Here's how the part is built. I have some questions about the finished solid (model axes, mm). Coordinates: 2 decimals unless noted, no trailing zeros. Loops run counter-clockwise (first coordinate to the right, second up) from the corner with the lowest first, then second, coordinate; pieces in that order, holes last. Notation, with made-up numbers: (-11.5, 55) - (25.5, 55) arc R11 cw to (25.5, 63) - close; hole circle Ø4 at (35, 77). An arc over 180 degrees is marked (long way). Use a Markdown table: item, result.
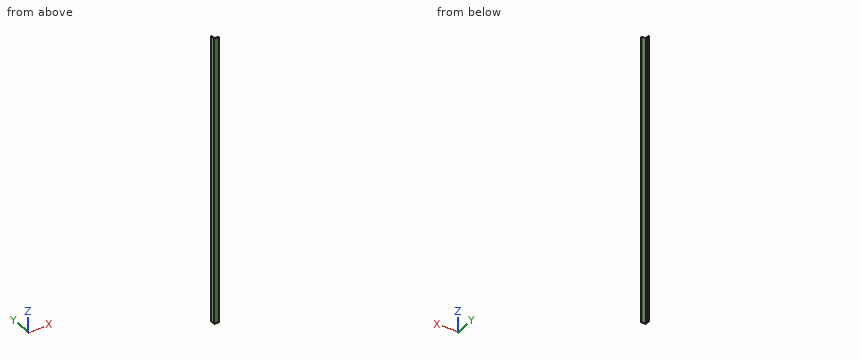
Autodesk Inventor part; units mm, degrees
ref_plane "Plano inicial" through (0, 0, 0) normal (0, 0, 1) x (1, 0, 0)
ref_plane "Plano final" through (0, 0, 2400) normal (0, 0, 1) x (1, 0, 0)
ref_plane "Plano de trabajo4" through (4.8672, 4.8672, 1401) normal (0, 0, 1) x (1, 0, 0)
ref_plane "Plano inicial" through (0, 0, 0) normal (0, 0, 1) x (1, 0, 0)
ref_plane "Plano final" through (0, 0, 2400) normal (0, 0, 1) x (1, 0, 0)
sketch "Boceto" plane through (0, 0, 0) normal (0, 0, 1) x (1, 0, 0)
  line L0 (38.1, 0) -> (0, 0)
  line L1 (0, 0) -> (0, 38.1)
  line L2 (0, 38.1) -> (2.4765, 38.1)
  line L3 (4.7625, 35.814) -> (4.7625, 9.5885)
  line L4 (9.5885, 4.7625) -> (35.814, 4.7625)
  line L5 (38.1, 2.4765) -> (38.1, 0)
  line L6 (0, -11.0414) -> (0, 31.5385) construction
  line L7 (-11.0414, 0) -> (31.5385, 0) construction
  arc A0 (4.7625, 9.5885) -> (9.5885, 4.7625) centre (9.5885, 9.5885) ccw
  arc A1 (4.7625, 35.814) -> (2.4765, 38.1) centre (2.4765, 35.814) ccw
  arc A2 (38.1, 2.4765) -> (35.814, 4.7625) centre (35.814, 2.4765) ccw
  line L8 (0, 48.4964) -> (0, -20.9644) construction
  line L9 (-20.9644, 0) -> (48.4964, 0) construction
  point P0 (4.7625, 38.1)
  point P1 (4.7625, 4.7625)
  point P2 (38.1, 4.7625)
  dimension "d0" = 38.1
  dimension "d1" = 38.1
  dimension "d2" = 4.7625
  dimension "d3" = 4.7625
  dimension "d10" = 0
  dimension "d11" = 0
  dimension "d14" = 4.826
  dimension "d15" = 2.286
extrude "Cuerpo" add sketch "Boceto" along normal up to surface (2400 mm away) from surface at 0
sketch "Sketch3" plane through (0, 0, 0) normal (0, 0, 1) x (1, 0, 0)
  line L0 (0, 0) -> (10, 0)
ref_plane "Work Plane3" through (0, 0, 0) normal (0, -1, 0) x (1, 0, 0)
sketch "Sketch4" plane through (0, 0, 0) normal (0, -1, 0) x (1, 0, 0)
  line L0 (-2, 0) -> (12, 0)
  line L1 (-2, 2400) -> (12, 2400)
  dimension "d17" = 2400
sketch "Boceto5" plane through (0, 0, 2400) normal (0, 0, 1) x (1, 0, 0)
  line L0 (0, 0) -> (0, 38.1)
  circle A0 centre (0, 0) radius 57.437
ref_plane "Plano de trabajo4" through (4.8672, 4.8672, 1401) normal (0, 0, 1) x (1, 0, 0)
equation "\"d0\" = G_H"
equation "\"d1\" = G_H"
equation "\"d2\" = G_T"
equation "\"d3\" = G_T"
equation "\"d14\" = G_IR"
equation "\"d15\" = G_ER"
equation "\"d4\" = G_L"
equation "\"G_H\" = 38.1"
equation "\"G_T\" = 4.7625"
equation "\"G_ER\" = 2.286"
equation "\"G_IR\" = 4.826"
equation "\"G_L\" = d17"
equation "\"ex\" = 0"
equation "\"G_OFFSET_START\" = 0"
equation "\"G_OFFSET_END\" = 0"
properties part number "AISC - L 1,5 x 1,5 x 3/16 - 94,488" material "Acero, suave"
Q1. Please list where these lines run through material, in increasing order: L1, parallel to Y at x = 26, z = 767.5; L2, parallel to X at y = 3, z = 264. Write a range as from..to.
Check values:
| item | result |
|---|---|
| L1 | 0..4.76 |
| L2 | 0..38.04 |
Q2. I want a section at A-A, the plane z = 681. Write out the boundary of the cut face in (x, y), then the cut area to 3 significant figures.
Check values:
| item | result |
|---|---|
| outline | (0, 0) - (38.1, 0) - (38.1, 2.48) arc R2.29 ccw to (35.81, 4.76) - (9.59, 4.76) arc R4.83 cw to (4.76, 9.59) - (4.76, 35.81) arc R2.29 ccw to (2.48, 38.1) - (0, 38.1) - close |
| area | 343 mm^2 |
Q3. I want a section at B-B, the plane x = 18. Write out the boundary of the cut face in (y, z).
Check values:
| item | result |
|---|---|
| outline | (0, 0) - (4.76, 0) - (4.76, 2400) - (0, 2400) - close |
Q4. Will these pins go through, and if not, where does the flat tip stop? P1, Ø8, axis at x = 16.5, z = 1236, coming from the +Y side; P2, Ø1.5, axis at y = 15, z = 1776, coming from the +X side.
Check values:
| item | result |
|---|---|
| P1 | y = 4.76 |
| P2 | x = 4.76 |
